Can you work these out from the model? Positions are in its coordinate system, mm. Face numbers are marked on the shaded views. A direction names the side the tool comes from. Give positions to 0.01 mm unless a question says otherwise; leave off trailing zeros. Order: outer loops, then holes, each group sorted by start corner. A loop starts at its lowest first (then second) coordinate and runs counter-clockwise, first axis right, second up. Notation, with made-up numbers: M -20,33.25 L 9,33.25 A6 cw 9,40.25 Z; hole C 65.5,-3 d10. An arc over 180 degrees is marked long. One line per question, with ' | ' between items. Start each with the question number.
1) I'm going to push flat-ended pins straight in: pin 1 Ø0.9 at (y, z) = (1.5, -32.5) entering from -X; pin 2 Ø11 at (x, y) = (-61, 36) entering from +Z; pin 3 Ø0.9 at (y, z) = (1.5, -30.5) entering from +X. Where does each tip first touch, or does it pass through?
2) If we section it at C-C, the plane y = 38: State how many separate pieces and enclosed holes the cut face has, plus the area to 3 significant figures.
3) If we section it at A-A, the plane y = 9.5: Please give me the cut outline in (x, z), plus the area to 3 significant figures.
4) Please list where these lines run through material, in increasing order: line 1 along X through (y, z) = (1.9, 31.5); line 2 along X through (y, z) = (40.9, 26.5) (3 decimals); line 3 along X through (y, z) = (42, 12). Write a range as [from, to].
5) For the marked faces 5 and 6, which set-ups out of +Z, -Z, +X, -X, +Y, -Y let a thin tool reach every point of the face, with its end or its side?
6) Thinking about a two-plate mould opening in Z: for the marked faces 1, 2, 3 and 4, which applies, +Z half, -Z half, draft (parallel to the pull), parting line (faces both ways), or undercut?
7) If we section it at B-B, the plane z = 26.5: Please give me the cut outline in (x, y) (3 decimals), plus the area to 3 significant figures.
8) If we section it at D-D, the plane z = -3: Please give me the cut outline in (x, y), plus the area to 3 significant figures.
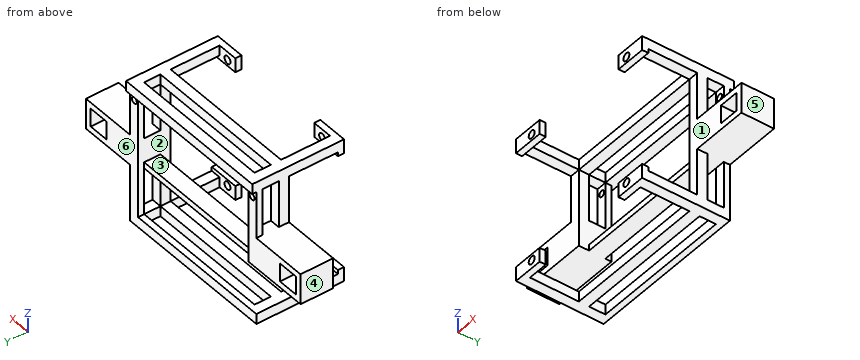
```python
from build123d import *

# Parameters (mm, degrees)
SKETCH1_W             = 15
SKETCH1_H             = 7
SKETCH1_R             = 1.9
BOSS_EXTRUDE1_DEPTH   = 3
BOSS_EXTRUDE1_2_DEPTH = 3
BOSS_EXTRUDE1_3_DEPTH = 3
BOSS_EXTRUDE1_4_DEPTH = 3
SKETCH2_W             = 5
SKETCH2_H             = 5
BOSS_EXTRUDE2_DEPTH   = 37
SKETCH4_W             = 5
SKETCH4_H             = 61
BOSS_EXTRUDE3_DEPTH   = 3
BOSS_EXTRUDE3_2_DEPTH = 3
SKETCH5_W             = 80
SKETCH5_H             = 5
BOSS_EXTRUDE5_DEPTH   = 3
SKETCH6_W             = 80
SKETCH6_H             = 5
BOSS_EXTRUDE6_DEPTH   = 5
SKETCH7_R             = 1.55
CUT_EXTRUDE1_DEPTH    = 3
SKETCH8_W             = 70
SKETCH8_H             = 5
BOSS_EXTRUDE7_DEPTH   = 5
SKETCH9_W             = 61
SKETCH9_H             = 5
BOSS_EXTRUDE8_DEPTH   = 5
SKETCH13_W            = 33
SKETCH13_H            = 15
SKETCH13_W_2          = 10
SKETCH13_H_2          = 9
BOSS_EXTRUDE10_DEPTH  = 16
SKETCH14_W            = 3
SKETCH14_H            = 8
BOSS_EXTRUDE11_DEPTH  = 70
SKETCH15_W            = 5
SKETCH15_H            = 23
CUT_EXTRUDE4_DEPTH    = 16


with BuildPart() as part:
    # Sketch1 → Boss-Extrude1 (new body)
    with BuildSketch(Plane(origin=(0, 0, 0), x_dir=(1, 0, 0), z_dir=(0, 1, 0))):
        with Locations((32.5, 32)):
            Rectangle(SKETCH1_W, SKETCH1_H)
        with Locations(Location((30, 31.5, 0), (0, 0, 270))):
            Circle(SKETCH1_R, mode=Mode.SUBTRACT)
    extrude(amount=BOSS_EXTRUDE1_DEPTH)



with BuildPart() as body_2:
    # Sketch1 → Boss-Extrude1 2 (new body)
    with BuildSketch(Plane(origin=(0, 0, 0), x_dir=(1, 0, 0), z_dir=(0, 1, 0))):
        with Locations((32.5, -32)):
            Rectangle(SKETCH1_W, SKETCH1_H)
        with Locations(Location((30, -31.5, 0), (0, 0, 90))):
            Circle(SKETCH1_R, mode=Mode.SUBTRACT)
    extrude(amount=BOSS_EXTRUDE1_2_DEPTH)


with BuildPart() as body_3:
    # Sketch1 → Boss-Extrude1 3 (new body)
    with BuildSketch(Plane(origin=(0, 0, 0), x_dir=(1, 0, 0), z_dir=(0, 1, 0))):
        with Locations((-32.5, -32)):
            Rectangle(SKETCH1_W, SKETCH1_H)
        with Locations(Location((-30, -31.5, 0), (0, 0, 270))):
            Circle(SKETCH1_R, mode=Mode.SUBTRACT)
    extrude(amount=BOSS_EXTRUDE1_3_DEPTH)


with BuildPart() as body_4:
    # Sketch1 → Boss-Extrude1 4 (new body)
    with BuildSketch(Plane(origin=(0, 0, 0), x_dir=(1, 0, 0), z_dir=(0, 1, 0))):
        with Locations((-32.5, 32)):
            Rectangle(SKETCH1_W, SKETCH1_H)
        with Locations(Location((-30, 31.5, 0), (0, 0, 90))):
            Circle(SKETCH1_R, mode=Mode.SUBTRACT)
    extrude(amount=BOSS_EXTRUDE1_4_DEPTH)


with BuildPart() as part_1:
    add(part.part)

    add(body_2.part)  # Boss-Extrude2 merges body 2

    add(body_3.part)  # Boss-Extrude2 merges body 3

    add(body_4.part)  # Boss-Extrude2 merges body 4
    # Sketch2 → Boss-Extrude2 (add)
    with BuildSketch(Plane(origin=(0, 3, 0), x_dir=(1, 0, 0), z_dir=(0, 1, 0))):
        with Locations((37.5, 33)):
            Rectangle(SKETCH2_W, SKETCH2_H)
        with Locations((37.5, -33)):
            Rectangle(SKETCH2_W, SKETCH2_H)
        with Locations((-37.5, -33)):
            Rectangle(SKETCH2_W, SKETCH2_H)
        with Locations((-37.5, 33)):
            Rectangle(SKETCH2_W, SKETCH2_H)
    extrude(amount=BOSS_EXTRUDE2_DEPTH)



with BuildPart() as body_2_2:
    # Sketch4 → Boss-Extrude3 (new body)
    with BuildSketch(Plane(origin=(0, 40, 0), x_dir=(1, 0, 0), z_dir=(0, 1, 0))):
        with Locations((37.5, 0)):
            Rectangle(SKETCH4_W, SKETCH4_H)
    extrude(amount=BOSS_EXTRUDE3_DEPTH)


with BuildPart() as body_3_2:
    # Sketch4 → Boss-Extrude3 2 (new body)
    with BuildSketch(Plane(origin=(0, 40, 0), x_dir=(1, 0, 0), z_dir=(0, 1, 0))):
        with Locations((-37.5, 0)):
            Rectangle(SKETCH4_W, SKETCH4_H)
    extrude(amount=BOSS_EXTRUDE3_2_DEPTH)


with BuildPart() as part_2:
    add(part_1.part)

    add(body_2_2.part)  # Boss-Extrude5 merges body 2 2

    add(body_3_2.part)  # Boss-Extrude5 merges body 3 2
    # Sketch5 → Boss-Extrude5 (add)
    with BuildSketch(Plane(origin=(0, 40, 0), x_dir=(1, 0, 0), z_dir=(0, 1, 0))):
        with Locations((0, 33)):
            Rectangle(SKETCH5_W, SKETCH5_H)
    extrude(amount=BOSS_EXTRUDE5_DEPTH)

    # Sketch6 → Boss-Extrude6 (add)
    with BuildSketch(Plane(origin=(0, 40, 0), x_dir=(1, 0, 0), z_dir=(0, 1, 0))):
        with Locations((0, -33)):
            Rectangle(SKETCH6_W, SKETCH6_H)
    extrude(amount=BOSS_EXTRUDE6_DEPTH)

    # Sketch7 → Cut-Extrude1 (cut)
    with BuildSketch(Plane(origin=(0, 43, 0), x_dir=(1, 0, 0), z_dir=(0, 1, 0))):
        with Locations(Location((-37.325, -26.5, 0), (0, 0, 270))):
            Circle(SKETCH7_R)
        with Locations(Location((37.325, -26.5, 0), (0, 0, 270))):
            Circle(SKETCH7_R)
    extrude(amount=-CUT_EXTRUDE1_DEPTH, mode=Mode.SUBTRACT)

    # Sketch8 → Boss-Extrude7 (add)
    with BuildSketch(Plane.XY.offset(35.5)):
        with Locations((0, 29.5)):
            Rectangle(SKETCH8_W, SKETCH8_H)
    boss_extrude7 = extrude(amount=-BOSS_EXTRUDE7_DEPTH)

    # Mirror1: Boss-Extrude7 across plane
    add(boss_extrude7.mirror(Plane.XY))

    # Sketch9 → Boss-Extrude8 (add)
    with BuildSketch(Plane(origin=(40, 0, 0), x_dir=(0, 0, -1), z_dir=(1, 0, 0))):
        with Locations((0, 29.5)):
            Rectangle(SKETCH9_W, SKETCH9_H)
    boss_extrude8 = extrude(amount=-BOSS_EXTRUDE8_DEPTH)

    # Mirror2: Boss-Extrude8 across plane
    add(boss_extrude8.mirror(Plane(origin=(0, 0, 0), x_dir=(0, 0, 1), z_dir=(1, 0, 0))))

    # Sketch13 → Boss-Extrude10 (add)
    with BuildSketch(Plane(origin=(0, 43, 0), x_dir=(1, 0, 0), z_dir=(0, 1, 0))):
        with Locations((51.5, 0)):
            Rectangle(SKETCH13_W, SKETCH13_H)
        with Locations((60, 0)):
            Rectangle(SKETCH13_W_2, SKETCH13_H_2, mode=Mode.SUBTRACT)
    boss_extrude10 = extrude(amount=-BOSS_EXTRUDE10_DEPTH)

    # Mirror3: Boss-Extrude10 across plane
    add(boss_extrude10.mirror(Plane(origin=(0, 0, 0), x_dir=(0, 0, 1), z_dir=(1, 0, 0))))

    # Sketch14 → Boss-Extrude11 (add)
    with BuildSketch(Plane(origin=(-35, 0, 0), x_dir=(0, 0, -1), z_dir=(1, 0, 0))):
        with Locations((6, 36)):
            Rectangle(SKETCH14_W, SKETCH14_H)
    extrude(amount=BOSS_EXTRUDE11_DEPTH)

    # Sketch15 → Cut-Extrude4 (cut)
    with BuildSketch(Plane(origin=(0, 43, 0), x_dir=(1, 0, 0), z_dir=(0, 1, 0))):
        with Locations((-37.5, 19)):
            Rectangle(SKETCH15_W, SKETCH15_H)
    extrude(amount=-CUT_EXTRUDE4_DEPTH, mode=Mode.SUBTRACT)


solid = part_2.part
```
Results found:
1) pin 1: stops at x = -40 | pin 2: stops at z = 7.5 | pin 3: stops at x = 40
2) separate pieces: 5 | enclosed holes: 2 | area: 1,120 mm²
3) outline: M -40,-35.5 L -35,-35.5 L -35,-30.5 L -40,-30.5 Z; M -40,30.5 L -35,30.5 L -35,35.5 L -40,35.5 Z; M 35,-35.5 L 40,-35.5 L 40,-30.5 L 35,-30.5 Z; M 35,30.5 L 40,30.5 L 40,35.5 L 35,35.5 Z | area: 100 mm²
4) line 1: x = [-40, -31.9], [-28.1, -25], [25, 28.1], [31.9, 40] | line 2: x = [-40, -38.875], [-35.775, -35], [35, 35.775], [38.875, 40] | line 3: x = [-40, -35], [35, 40]
5) face 5: +Z, -Z, +X, +Y, -Y | face 6: -Z, +X, -X, +Y
6) face 1: undercut | face 2: undercut | face 3: +Z half | face 4: draft
7) outline: M -40,27 L -35,27 L -35,32 L -40,32 Z; M -40,40 L -38.875,40 L -38.875,43 L -40,43 Z; M -35.775,40 L -35,40 L -35,43 L -35.775,43 Z; M 35,27 L 40,27 L 40,32 L 35,32 Z; M 35,40 L 35.775,40 L 35.775,43 L 35,43 Z; M 38.875,40 L 40,40 L 40,43 L 38.875,43 Z | area: 61.4 mm²
8) outline: M -68,27 L -65,27 L -65,43 L -68,43 Z; M -55,27 L -35,27 L -35,43 L -55,43 Z; M 35,27 L 55,27 L 55,43 L 35,43 Z; M 65,27 L 68,27 L 68,43 L 65,43 Z | area: 736 mm²
